```python
from build123d import *

# Parameters (mm, degrees)
SKETCH1_R           = 20
BOSS_EXTRUDE1_DEPTH = 5
SKETCH2_R           = 12.5
BOSS_EXTRUDE2_DEPTH = 5
SKETCH3_R           = 20
BOSS_EXTRUDE3_DEPTH = 5
SKETCH4_R           = 12.5
BOSS_EXTRUDE4_DEPTH = 5
SKETCH5_R           = 20
BOSS_EXTRUDE5_DEPTH = 5
FILLET1_R           = 1
SKETCH6_R           = 1.6
CUT_EXTRUDE1_DEPTH  = 25


with BuildPart() as part:
    # Sketch1 → Boss-Extrude1 (new body)
    with BuildSketch(Plane(origin=(0, 0, 0), x_dir=(0, 0, -1), z_dir=(1, 0, 0))):
        Circle(SKETCH1_R)
    extrude(amount=BOSS_EXTRUDE1_DEPTH)

    # Sketch2 → Boss-Extrude2 (add)
    with BuildSketch(Plane(origin=(5, 0, 0), x_dir=(0, 0, -1), z_dir=(1, 0, 0))):
        Circle(SKETCH2_R)
    extrude(amount=BOSS_EXTRUDE2_DEPTH)

    # Sketch3 → Boss-Extrude3 (add)
    with BuildSketch(Plane(origin=(10, 0, 0), x_dir=(0, 0, -1), z_dir=(1, 0, 0))):
        Circle(SKETCH3_R)
    extrude(amount=BOSS_EXTRUDE3_DEPTH)

    # Sketch4 → Boss-Extrude4 (add)
    with BuildSketch(Plane(origin=(15, 0, 0), x_dir=(0, 0, -1), z_dir=(1, 0, 0))):
        Circle(SKETCH4_R)
    extrude(amount=BOSS_EXTRUDE4_DEPTH)

    # Sketch5 → Boss-Extrude5 (add)
    with BuildSketch(Plane(origin=(20, 0, 0), x_dir=(0, 0, -1), z_dir=(1, 0, 0))):
        Circle(SKETCH5_R)
    extrude(amount=BOSS_EXTRUDE5_DEPTH)

    # Fillet1
    fillet1_edges = [part.edges().sort_by_distance(p)[0] for p in [
        (25, 0, 20),
        (0, 0, 20),
    ]]
    fillet(fillet1_edges, radius=FILLET1_R)

    # Sketch6 → Cut-Extrude1 (cut)
    with BuildSketch(Plane(origin=(25, 0, 0), x_dir=(0, 0, -1), z_dir=(1, 0, 0))):
        Circle(SKETCH6_R)
    extrude(amount=-CUT_EXTRUDE1_DEPTH, mode=Mode.SUBTRACT)


solid = part.part
```
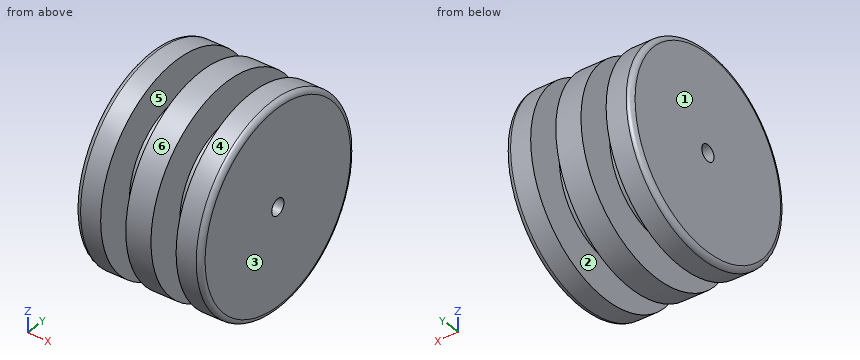
Design review of the part built by this model. Coordinates are the model's own, in mm. Face numbers are marked on the shaded views. A direction names the side the tool comes from. Give positions to 0.01 mm unless a question says otherwise; leave off trailing zeros. Write each loop counter-clockwise with the first axis right and the second up, starting at its lowest first coordinate (ties: lowest second). Pieces come first, ordered by that corner, then holes.
(1) Add section C-C (x = 11.75). Give the boundary of the cut face in (y, z).
Checked values:
outline: circle Ø40 at (0, 0); hole circle Ø3.2 at (0, 0)
(2) Tool access review of the marked faces 5 and 6: name each direction out of +Z, -Z, +X, -X, +Y, -Y from which nothing blocks a thin tool from reaching the whole face with its end or side.
Checked values:
face 5: none
face 6: +X, -X
(3) Clearance check with flat-ended pins moving along their axes: pin 1 Ø10 at (x, z) = (7, 4) entering from +Y; pin 2 Ø5 at (x, z) = (18.5, 12.5) entering from -Y; pin 3 Ø12 at (x, y) = (5.5, -10) entering from -Z. State where each tip first meets the part, or that it passes through.
Checked values:
pin 1: stops at y = 20
pin 2: stops at y = -17.02
pin 3: stops at z = -19.59
(4) Add section A-A (z = 0). Give the boundary of the cut face in (x, y), and give its area (3 significant figures).
Checked values:
outline: (0, -19) arc R1 ccw to (1, -20) - (5, -20) - (5, -12.5) - (10, -12.5) - (10, -20) - (15, -20) - (15, -12.5) - (20, -12.5) - (20, -20) - (24, -20) arc R1 ccw to (25, -19) - (25, -1.6) - (0, -1.6) - close; (0, 1.6) - (25, 1.6) - (25, 19) arc R1 ccw to (24, 20) - (20, 20) - (20, 12.5) - (15, 12.5) - (15, 20) - (10, 20) - (10, 12.5) - (5, 12.5) - (5, 20) - (1, 20) arc R1 ccw to (0, 19) - close
area: 769 mm2
(5) Wall thickness on line 1 along X through (y, z) = (-13, 9.5); line 2 along Y through (x, z) = (6.25, 0); line 3 along X through (y, z) = (16.5, -10.5): over which ranges is each line inside the solid? List them lowest first.
Checked values:
line 1: x = 0 to 5, 10 to 15, 20 to 25
line 2: y = -12.5 to -1.6, 1.6 to 12.5
line 3: x = 0.17 to 5, 10 to 15, 20 to 24.83
(6) Add section D-D (x = 18.75). Give the boundary of the cut face in (y, z).
Checked values:
outline: circle Ø25 at (0, 0); hole circle Ø3.2 at (0, 0)
(7) Mouldability with a two-part tool opening along X and no side actions: class the marked faces 1, 2, 3 and 4 as +X half, -X half, draft (parallel to the pull), parting line (faces both ways), or undercut.
Checked values:
face 1: -X half
face 2: undercut
face 3: +X half
face 4: draft
